from build123d import *

# Parameters (mm, degrees)
SKETCH_W        = 14
SKETCH_H        = 2
PAD_DEPTH       = 3.25
SKETCH001_W     = 22
SKETCH001_H     = 70
POCKET_DEPTH    = 2
POCKET001_DEPTH = 2.5
POCKET002_DEPTH = 3.001
CHAMFER_SIZE    = 1.99
CHAMFER001_SIZE = 1.99
FILLET_R        = 2.99


with BuildPart() as part:
    # Sketch → Pad (new body, symmetric)
    with BuildSketch(Plane.XZ):
        Polygon((-26, 0), (-26, 3), (-11, 3), (-11, 70), (11, 70), (11, 3), (26, 3), (26, 0), align=None)
        with Locations((0, 6)):
            Rectangle(SKETCH_W, SKETCH_H, mode=Mode.SUBTRACT)
    extrude(amount=PAD_DEPTH, both=True)

    # Sketch001 (on Face14 of Pad) → Pocket (cut)
    with BuildSketch(Plane.XZ.offset(3.25)):
        with Locations((0, 38)):
            Rectangle(SKETCH001_W, SKETCH001_H)
    extrude(amount=-POCKET_DEPTH, mode=Mode.SUBTRACT)

    # Sketch002 (on Face16 of Pocket) → Pocket001 (cut)
    with BuildSketch(Plane.XZ.offset(1.25)):
        Polygon((-10, 68.5), (10, 68.5), (10, 12.5), (7, 12.5), (7, 7), (-7, 7), (-7, 12.5), (-10, 12.5), align=None)
    extrude(amount=-POCKET001_DEPTH, mode=Mode.SUBTRACT)

    # Sketch003 (on Face3 of Pocket001) → Pocket002 (cut, through all)
    with BuildSketch(Plane(origin=(0, 0, 3), x_dir=(-1, 0, 0), z_dir=(0, 0, 1))):
        with BuildLine():
            ThreePointArc((-19.59, -1.65), (-17.94, 0), (-19.59, 1.65))
            Line((-19.59, 1.65), (-21.59, 1.65))
            ThreePointArc((-21.59, 1.65), (-23.24, 0), (-21.59, -1.65))
            Line((-19.59, -1.65), (-21.59, -1.65))
        make_face()
        with BuildLine():
            ThreePointArc((19.59, 1.65), (17.94, 0), (19.59, -1.65))
            Line((19.59, -1.65), (21.59, -1.65))
            ThreePointArc((21.59, -1.65), (23.24, 0), (21.59, 1.65))
            Line((19.59, 1.65), (21.59, 1.65))
        make_face()
    extrude(amount=-POCKET002_DEPTH, mode=Mode.SUBTRACT)

    # Chamfer
    chamfer_edges = [part.edges().sort_by_distance(p)[0] for p in [
        (0, -1.25, 3),
    ]]
    chamfer(chamfer_edges, length=CHAMFER_SIZE)

    # Chamfer001
    chamfer001_edges = [part.edges().sort_by_distance(p)[0] for p in [
        (-11, 1, 3),
        (11, 1, 3),
    ]]
    chamfer(chamfer001_edges, length=CHAMFER001_SIZE)

    # Fillet
    fillet_edges = [part.edges().sort_by_distance(p)[0] for p in [
        (-26, 3.25, 1.5),
        (-26, -3.25, 1.5),
        (26, -3.25, 1.5),
        (26, 3.25, 1.5),
    ]]
    fillet(fillet_edges, radius=FILLET_R)


solid = part.part
The model under review builds one solid part; all positions refer to its coordinate system, in mm. A direction names the side the tool comes from. Coordinates: 2 decimals unless noted, no trailing zeros. Write each loop counter-clockwise with the first axis right and the second up, starting at its lowest first coordinate (ties: lowest second). Pieces come first, ordered by that corner, then holes. Notation, with made-up numbers: (49, 83.25) -> (86, 83.25) arc R8 ccw to (86, 90.25) -> close; hole circle Ø9 at (71.5, 80). An arc over 180 degrees is marked (long way). Answer in a Markdown table with one row per item.
1. Draft analysis for pull direction X (two halves, no side actions). For faces 5 (the flat face through (0, 1, 70)), 6 (the flat face through (9, 0, 12.5)), 7 (the cylindrical face through (-25.1, -2.4, 1.5)), state which applies: +X half, -X half, draft (parallel to the pull), parting line (faces both ways), or undercut.
Answers below:
| item | result |
|---|---|
| face 5 | draft |
| face 6 | undercut |
| face 7 | -X half |
2. Clearance check with flat-ended pins moving along their axes: pin 1 Ø5 at (x, z) = (3, 12.5) entering from -Y; pin 2 Ø0.8 at (y, z) = (0, 41) entering from -X; pin 3 Ø24 at (x, z) = (-1.5, 50) entering from -Y. State where each tip first meets the part, or that it passes through.
Answers below:
| item | result |
|---|---|
| pin 1 | stops at y = 1.25 |
| pin 2 | stops at x = -11 |
| pin 3 | stops at y = -1.25 |
3. Wall thickness on probe 1 along X at (y, z) = (-0.25, 16); probe 2 along X at (y, z) = (0.25, 8); probe 3 along Z at (x, y) = (-5.5, 2): over which ranges is each line inside the solid? List them lowest first. Write a range as [from, to].
Answers below:
| item | result |
|---|---|
| probe 1 | x = [-11, -10], [10, 11] |
| probe 2 | x = [-11, -7], [7, 11] |
| probe 3 | z = [0, 5], [7, 70] |
4. For faces 1 (the flat face through (-10, 0, 40)), 2 (the flat face through (-10.6, -1.25, 40.1)), 3 (the cylindrical face through (23.24, -0.04, 1.52)), 4 (the flat face through (0, 1, 5)), list the 3-axis set-ups (+Z, -Z, +X, -X, +Y, -Y) from which the entire face can be reached by the end or side of a thin tool; tool diameter is ignored.
Answers below:
| item | result |
|---|---|
| face 1 | -Y |
| face 2 | +Z, +X, -X, -Y |
| face 3 | +Z, -Z |
| face 4 | +Y, -Y |
5. We need section C-C, the plane y = -2.5. State the section outline as (x, z) points.
Answers below:
| item | result |
|---|---|
| outline | (-24.99, 0) -> (24.99, 0) -> (24.99, 3) -> (12.99, 3) -> (12.25, 3.74) -> (-12.25, 3.74) -> (-12.99, 3) -> (-24.99, 3) -> close |
6. We need section B-B, the plane z = 45. State the section outline as (x, y) points.
Answers below:
| item | result |
|---|---|
| outline | (-11, -1.25) -> (-10, -1.25) -> (-10, 1.25) -> (10, 1.25) -> (10, -1.25) -> (11, -1.25) -> (11, 3.25) -> (-11, 3.25) -> close |
